Input: part model. Units: mm. Frame: model coordinates. A direction names the side the tool comes from. Coordinates: 2 decimals unless noted, no trailing zeros. Loops run counter-clockwise (first coordinate to the right, second up) from the corner with the lowest first, then second, coordinate; pieces in that order, holes last. Notation, with made-up numbers: M 78.25,82.25 L 115.25,82.25 A25 ccw 115.25,109.25 Z; hole C 85,56.25 d7. An arc over 180 degrees is marked long. Use a Markdown table: item, result. Add a question column.
1. Section A-A on z = 38. Output: boundary loops of the cut face in (x, y), then the cut area to 3 significant figures.
2. Section C-C on y = -5. State how many separate pieces and enclosed holes the cut face has, then the cut area to 3 significant figures.
3. Section B-B on x = 100. Output: boundary loops of the cut face in (y, z), then the cut area to 3 significant figures.
4. Pin query (flat end, axial travel): pin 1 (3 mm diameter, centred on x = 14, y = -2, fed in from +Z); pin 2 (2 mm diameter, centred on y = -3.5, z = 13, fed in from +X); pin 3 (1.1 mm diameter, centred on y = -3.5, z = 17.5, fed in from -X). Return the tip coordinate at first contact, or that it passes through.
5. Draft query along X for faces 6 (the flat face through (65, -3, 55)), 7 (the flat face through (57.5, -3, 58)), 8 (the flat face through (128, -3, 61.35)), 9 (the flat face through (22.5, -3, 58)). Return one class per face: +X half, -X half, draft (parallel to the pull), parting line (faces both ways), or undercut.
6. Set-up query: faces 1 (the flat face through (15, -3, 3)), 2 (the cylindrical face through (163.5, -3.13, 47.22)), 3 (the flat face through (177, -3, 45)), 4 (the flat face through (132.5, -3, 58)), 5 (the flat face through (6.35, -3, 40)). Return all of +Z, -Z, +X, -X, +Y, -Y with unobstructed straight access to the full face (end or side cutting, diameter ignored); none if empty.
7. Line query: L1, parallel to Z at x = 45, y = -4.75; L2, parallel to X at y = -2.75, z = 18. Output: solid intervals per line, ascending. Write a range as [from, to].
8. Section D-D on z = 26.5. Output: boundary loops of the cut face in (x, y).
```python
from build123d import *

# Parameters (mm, degrees)
F1_DEPTH = 6.35


with BuildPart() as f1:
    # F0 (on Front) → F1 (new body)
    with BuildSketch(Plane.XZ):
        Polygon((0, 10), (0, 0), (15, 0), (15, 6.35), (18.5, 6.35), (18.5, 14), (17.3, 14), (17.3, 16.27), (18.5, 16.27), (18.5, 20), (21.5, 20), (21.5, 16.27), (22.7, 16.27), (22.7, 14), (21.5, 14), (21.5, 6.35), (25, 6.35), (25, 0), (155, 0), (155, 6.35), (158.5, 6.35), (158.5, 14), (157.3, 14), (157.3, 16.27), (158.5, 16.27), (158.5, 20), (161.5, 20), (161.5, 16.27), (162.7, 16.27), (162.7, 14), (161.5, 14), (161.5, 6.35), (165, 6.35), (165, 0), (180, 0), (180, 10), (173.65, 10), (173.65, 20), (180, 20), (180, 35), (173.65, 35), (173.65, 45), (180, 45), (180, 55), (157.5, 55), (157.5, 61.35), (147.5, 61.35), (147.5, 55), (132.5, 55), (132.5, 61.35), (122.5, 61.35), (122.5, 55), (107.5, 55), (107.5, 61.35), (97.5, 61.35), (97.5, 55), (82.5, 55), (82.5, 61.35), (72.5, 61.35), (72.5, 55), (57.5, 55), (57.5, 61.35), (47.5, 61.35), (47.5, 55), (32.5, 55), (32.5, 61.35), (22.5, 61.35), (22.5, 55), (0, 55), (0, 45), (6.35, 45), (6.35, 35), (0, 35), (0, 20), (6.35, 20), (6.35, 10), align=None)
        with BuildLine():
            ThreePointArc((35, 12.3), (36.464466, 15.835534), (40, 17.3))
            Line((40, 17.3), (140, 17.3))
            ThreePointArc((140, 17.3), (143.535534, 15.835534), (145, 12.3))
            Line((145, 12.3), (145, 11.35))
            ThreePointArc((145, 11.35), (143.535534, 7.814466), (140, 6.35))
            Line((140, 6.35), (40, 6.35))
            ThreePointArc((40, 6.35), (36.464466, 7.814466), (35, 11.35))
            Line((35, 11.35), (35, 12.3))
        make_face(mode=Mode.SUBTRACT)
        with BuildLine():
            ThreePointArc((15, 43.65), (16.464466, 47.185534), (20, 48.65))
            Line((20, 48.65), (160, 48.65))
            ThreePointArc((160, 48.65), (163.535534, 47.185534), (165, 43.65))
            Line((165, 43.65), (165, 28.65))
            ThreePointArc((165, 28.65), (163.535534, 25.114466), (160, 23.65))
            Line((160, 23.65), (20, 23.65))
            ThreePointArc((20, 23.65), (16.464466, 25.114466), (15, 28.65))
            Line((15, 28.65), (15, 43.65))
        make_face(mode=Mode.SUBTRACT)
    extrude(amount=F1_DEPTH)


solid = f1.part
```
Answers below:
| question | item | result |
|---|---|---|
| 1 | outline | M 6.35,-6.35 L 15,-6.35 L 15,0 L 6.35,0 Z; M 165,-6.35 L 173.65,-6.35 L 173.65,0 L 165,0 Z |
| 1 | area | 110 mm² |
| 2 | separate pieces | 1 |
| 2 | enclosed holes | 2 |
| 2 | area | 4,900 mm² |
| 3 | outline | M -6.35,0 L 0,0 L 0,6.35 L -6.35,6.35 Z; M -6.35,17.3 L 0,17.3 L 0,23.65 L -6.35,23.65 Z; M -6.35,48.65 L 0,48.65 L 0,61.35 L -6.35,61.35 Z |
| 3 | area | 161 mm² |
| 4 | pin 1 | stops at z = 55 |
| 4 | pin 2 | stops at x = 173.65 |
| 4 | pin 3 | stops at x = 6.35 |
| 5 | face 6 | undercut |
| 5 | face 7 | undercut |
| 5 | face 8 | draft |
| 5 | face 9 | -X half |
| 6 | face 1 | -Z, +Y, -Y |
| 6 | face 2 | +Y, -Y |
| 6 | face 3 | +X, +Y, -Y |
| 6 | face 4 | +Z, +Y, -Y |
| 6 | face 5 | -X, +Y, -Y |
| 7 | L1 | z = [0, 6.35], [17.3, 23.65], [48.65, 55] |
| 7 | L2 | x = [6.35, 18.5], [21.5, 158.5], [161.5, 173.65] |
| 8 | outline | M 0,-6.35 L 15.49,-6.35 L 15.49,0 L 0,0 Z; M 164.51,-6.35 L 180,-6.35 L 180,0 L 164.51,0 Z |
